Source: CAD feature listing. Evaluate the final solid. Frame: model axes, mm. A direction names the side the tool comes from. Give positions to 0.01 mm unless a question says otherwise; leave off trailing zeros. Loops run counter-clockwise (first coordinate to the right, second up) from the corner with the lowest first, then second, coordinate; pieces in that order, holes last. Notation, with made-up numbers: (76.5, 34.25) - (94.5, 34.25) arc R30 cw to (94.5, 58.25) - close; hole circle Ø7 at (64, 88.25). An arc over 180 degrees is marked (long way). Write each question's results on one line, items separated by ' | '. Start each with the question number.
(1) Pull-direction query (Z, two-part tool) for faces 4 (the cylindrical face through (70.33, -16.94, 0.11)), 5 (the cylindrical face through (79, -13, 0)), 6 (the cylindrical face through (10.726, -4.056, -8.644)); classes: pulls with the +Z half, pulls with the -Z half, needs draft (parallel to the pull), parting line crosses it, or undercut.
(2) Cut plane B-B on y = -6. Return the cut outline in (x, z), then the cut area to 3 significant figures.
(3) Reachability of faces 1 (the flat face through (46, -8, 8)), 2 (the flat face through (45, -8, -8)), 3 (the flat face through (78.8, -9, 0.1)) from +Z, -Z, +X, -X, +Y, -Y: full face, straight path, thin tool, end or side. Return the list, or none.
(4) Contact query for flat-ended pins moving along their axis: pin 1 (5 mm diameter, centred on x = 53, y = -11, fed in from -Z); pin 2 (10 mm diameter, centred on x = 57, z = -2, fed in from +Y); pin 3 (10 mm diameter, centred on x = 28, z = 5.5, fed in from +Y). Output: stop coordinate, or through.
(5) Cut plane D-D on y = -12.75. Return the cut outline in (x, z).
(6) Cut plane A-A on x = 0. Return the cut outline in (y, z).
(7) Cut plane C-C on x = 85. Return the cut outline in (y, z).
(8) Material intervals for line 1 along Z through (x, y) = (0, -2.75); line 2 along Z through (x, y) = (85, -15.25); line 3 along Y through (x, z) = (76.5, -6.5), sorted ascending. Write a range as [from, to].
from build123d import *

# Parameters (mm, degrees)
F0_R     = 6
F1_DEPTH = 25
F3_DEPTH = 12.5
F4_R     = 15


with BuildPart() as f1:
    # F0 (on Front) → F1 (new body)
    with BuildSketch(Plane.XZ):
        with BuildLine():
            ThreePointArc((9.604686, -8), (11.753905, -4.253905), (12.5, 0))
            ThreePointArc((12.5, 0), (11.753905, 4.253905), (9.604686, 8))
            ThreePointArc((9.604686, 8), (-12.5, 0), (9.604686, -8))
        make_face()
        Circle(F0_R, mode=Mode.SUBTRACT)
        with BuildLine():
            ThreePointArc((9.604686, 8), (11.753905, 4.253905), (12.5, 0))
            ThreePointArc((12.5, 0), (11.753905, -4.253905), (9.604686, -8))
            Line((9.604686, -8), (79, -8))
            ThreePointArc((79, -8), (75, 0), (79, 8))
            Line((79, 8), (9.604686, 8))
        make_face()
        with BuildLine():
            ThreePointArc((95, 0), (89.472136, 8.944272), (79, 8))
            ThreePointArc((79, 8), (75, 0), (79, -8))
            ThreePointArc((79, -8), (89.472136, -8.944272), (95, 0))
        make_face()
        with Locations((85, 0)):
            Circle(F0_R, mode=Mode.SUBTRACT)
    extrude(amount=F1_DEPTH)

    # F2 (on Top) → F3 (intersect, symmetric)
    with BuildSketch(Plane.XY):
        Polygon((20, 0), (-12.5, 0), (-12.5, -8), (19.300091, -8), (70.341622, -16.999999), (95, -16.999999), (95, -8.999999), (71.041532, -8.999999), align=None)
    extrude(amount=F3_DEPTH, both=True, mode=Mode.INTERSECT)

    # F4
    f4_edges = [f1.edges().sort_by_distance(p)[0] for p in [
        (20, 0, 0),
        (19.300091, -8, 0),
        (70.341622, -16.999999, 0),
        (71.041532, -8.999999, 0),
        (79, -12.999999, -8),
        (9.604686, -4, -8),
        (9.604686, -4, 8),
        (79, -12.999999, 8),
    ]]
    fillet(f4_edges, radius=F4_R)


solid = f1.part
Ans:
1) face 4: needs draft | face 5: undercut | face 6: pulls with the -Z half
2) outline: (6.85, -10.45) arc R15 cw to (15.07, -8) - (54.03, -8) - (54.03, 8) - (15.07, 8) arc R15 cw to (6.85, 10.45) arc R12.5 ccw (long way) to start; hole circle Ø12 at (0, 0) | area: 1,060 mm^2
3) face 1: +Z, +Y, -Y | face 2: -Z, +Y, -Y | face 3: +Z, -Z, +X, +Y
4) pin 1: z = -8 | pin 2: y = -5.64 | pin 3: y = -0.53
5) outline: (46.24, -8) - (75.2, -8) arc R15 cw to (81.08, -9.2) arc R10 ccw (long way) to (81.08, 9.2) arc R15 cw to (75.2, 8) - (46.24, 8) - close; hole circle Ø12 at (85, 0)
6) outline: (-8, -12.5) - (0, -12.5) - (0, -6) - (-8, -6) - close; (-8, 6) - (0, 6) - (0, 12.5) - (-8, 12.5) - close
7) outline: (-17, -10) - (-9, -10) - (-9, -6) - (-17, -6) - close; (-17, 6) - (-9, 6) - (-9, 10) - (-17, 10) - close
8) line 1: [-12.5, -6], [6, 12.5] | line 2: [-10, -6], [6, 10] | line 3: [-17, -9]
